Source: CAD feature listing. Evaluate the final solid. Frame: model axes, mm. Face numbers are marked on the shaded views. Round coordinates to 2 decimals unless told otherwise and drop trailing zeros. Order: outer loops, then holes, each group sorted by start corner. A loop starts at its lowest first (then second) coordinate and runs counter-clockwise, first axis right, second up. Notation, with made-up numbers: (86, 29) -> (98, 29) arc R22 cw to (98, 45) -> close; hole circle Ø5 at (-37.5, -23.5). An arc over 180 degrees is marked (long way). One line per item, written item: value. Start each with the question number.
1) Section D-D (z = -17). Return the cut outline in (x, y).
2) Mould query, pull axis X, two halves, no side actions, for the marked faces 1, 2 and 3. Classes: pulls with the +X half, pulls with the -X half, needs draft (parallel to the pull), parting line crosses it, or undercut.
3) Ray query, L1, parallel to Y at x = 24, z = 7; L2, parallel to X at y = 7.25, z = -13.5; L3, parallel to X at y = 5.75, z = -9.5. Return the intervals inside material, ascending.
4) Section A-A (z = 0). Return the cut outline in (x, y).
5) Section C-C (x = 15.5). Return the cut outline in (y, z).
6) Section B-B (x = 0). Return the cut outline in (y, z).
7) Pin query (flat end, axial travel): P1, Ø1.5, axis at y = -0.5, z = -6.5, coming from the -X side; P2, Ø5, axis at x = -4.5, y = 7.5, coming from the +Z side; P3, Ø1, axis at x = 3.5, y = -0.5, coming from the -Z side. Return the tip coordinate at first contact, or that it passes through.
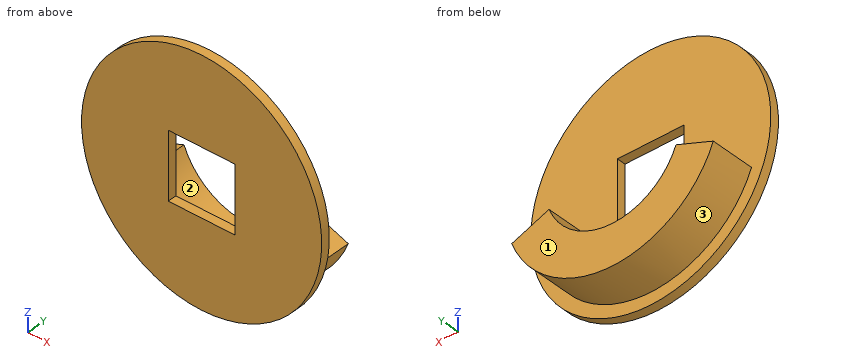
```python
from build123d import *

# Parameters (mm, degrees)
BOSS_EXTRUDE1_DEPTH = 10
SKETCH2_R           = 27
SKETCH2_W           = 15
SKETCH2_H           = 15
BOSS_EXTRUDE2_DEPTH = 2


with BuildPart() as part:
    # Sketch1 → Boss-Extrude1 (new body)
    with BuildSketch(Plane(origin=(0, 0, 0), x_dir=(1, 0, 0), z_dir=(0, 1, 0))):
        with BuildLine():
            Line((-22.669793675, 8.750454545), (-14.273573795, 5.509545455))
            ThreePointArc((-14.273573795, 5.509545455), (0, 15.3), (14.273573795, 5.509545455))
            Line((14.273573795, 5.509545455), (22.669793675, 8.750454545))
            ThreePointArc((22.669793675, 8.750454545), (0, 24.3), (-22.669793675, 8.750454545))
        make_face()
    extrude(amount=BOSS_EXTRUDE1_DEPTH)

    # Sketch2 → Boss-Extrude2 (add)
    with BuildSketch(Plane.XZ):
        with Locations(Location((0, 0, 0), (0, 0, 270))):
            Circle(SKETCH2_R)
        Rectangle(SKETCH2_W, SKETCH2_H, mode=Mode.SUBTRACT)
    extrude(amount=BOSS_EXTRUDE2_DEPTH)


solid = part.part
```
Findings:
1. outline: (-20.98, -2) -> (20.98, -2) -> (20.98, 0) -> (17.36, 0) -> (17.36, 10) -> (-17.36, 10) -> (-17.36, 0) -> (-20.98, 0) -> close
2. face 1: needs draft
2. face 2: undercut
2. face 3: parting line crosses it
3. L1: -2 to 0
3. L2: -20.2 to -7.2, 7.2 to 20.2
3. L3: -22.37 to -11.99, 11.99 to 22.37
4. outline: (-27, -2) -> (-7.5, -2) -> (-7.5, 0) -> (-27, 0) -> close; (7.5, -2) -> (27, -2) -> (27, 0) -> (7.5, 0) -> close
5. outline: (-2, -22.11) -> (0, -22.11) -> (0, -18.71) -> (10, -18.71) -> (10, -5.98) -> (0, -5.98) -> (0, 22.11) -> (-2, 22.11) -> close
6. outline: (-2, -27) -> (0, -27) -> (0, -24.3) -> (10, -24.3) -> (10, -15.3) -> (0, -15.3) -> (0, -7.5) -> (-2, -7.5) -> close; (-2, 7.5) -> (0, 7.5) -> (0, 27) -> (-2, 27) -> close
7. P1: x = -26.38
7. P2: z = -13.6
7. P3: z = -26.83
